Check sheet for the modelled part. Datum: model origin and axes. Units: mm. Face numbers are marked on the shaded views. A direction names the side the tool comes from. Give positions to 0.01 mm unless a question says otherwise; leave off trailing zeros. One line per item, written item: value. Start each with the question number.
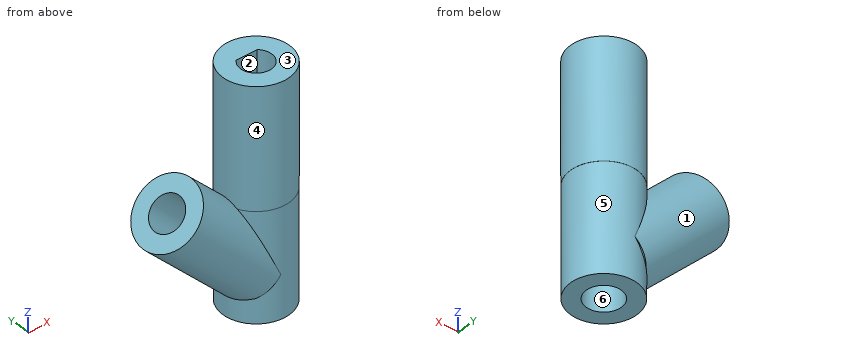
from build123d import *

# Parameters (mm, degrees)
SKETCH841_R     = 5.575015
PAD364_DEPTH    = 20
SKETCH842_R     = 5.560307
PAD365_DEPTH    = 18
SKETCH843_R     = 5.579276
PAD366_DEPTH    = 20
SKETCH844_R     = 2.85
POCKET224_DEPTH = 20
SKETCH845_R     = 2.95
POCKET225_DEPTH = 18.001


with BuildPart() as part:
    # Sketch841 → Pad364 (new body)
    with BuildSketch(Plane.XY):
        Circle(SKETCH841_R)
        with BuildLine():
            ThreePointArc((-1.794436, 1.881489), (0, -2.6), (1.794436, 1.881489))
            Line((-1.794436, 1.881489), (1.794436, 1.881489))
        make_face(mode=Mode.SUBTRACT)
    extrude(amount=PAD364_DEPTH)

    # Sketch842 → Pad365 (join)
    with BuildSketch(Plane.XY):
        Circle(SKETCH842_R)
    extrude(amount=-PAD365_DEPTH)

    # Sketch843 → Pad366 (join)
    with BuildSketch(Plane(origin=(-9, 0, 9), x_dir=(0.707107, 0, 0.707107), z_dir=(-0.707107, 0, 0.707107))):
        with Locations((-8.742249, 0)):
            Circle(SKETCH843_R)
    extrude(amount=-PAD366_DEPTH)

    # Sketch844 → Pocket224 (cut)
    with BuildSketch(Plane(origin=(-9, 0, 9), x_dir=(0.707107, 0, 0.707107), z_dir=(-0.707107, 0, 0.707107))):
        with Locations((-8.742247, 0)):
            Circle(SKETCH844_R)
    extrude(amount=-POCKET224_DEPTH, mode=Mode.SUBTRACT)

    # Sketch845 → Pocket225 (cut, through all)
    with BuildSketch(Plane.XY):
        Circle(SKETCH845_R)
    extrude(amount=-POCKET225_DEPTH, mode=Mode.SUBTRACT)


with BuildPart() as part_1:
    # Body064 placement: moved
    add(part.part.moved(Location((-52, -108, 0))))


solid = part_1.part
1) Cross-section at B-B (y = -108.5). State how many separate pieces and enclosed holes the cut face has, plus the area to 3 significant figures.
2) Gauge pin test, flat ends, axial feed: pin 1 (5.5 mm diameter, centred on x = -52, y = -108, fed in from -Z); pin 2 (1.5 mm diameter, centred on x = -60.5, z = -9, fed in from -Y); pin 3 (1 mm diameter, centred on x = -67, z = -1, fed in from -Y). Record the tip position at first contact, or that the pin passes through.
3) Draft check along Y on the marked faces 1, 2 and 3. Enter one of: released by +Y, released by -Y, zero draft, split by the parting line, or undercut.
4) Tool access check on the marked faces 4, 5 and 6. Record the directions out of +Z, -Z, +X, -X, +Y, -Y that give a thin tool (end or side, any length) a straight path to the whole face; none if there is none.
5) Material ranges on L1, parallel to Y at x = -52, z = -5; L2, parallel to X at y = -108, z = 9; L3, parallel to Y at x = -63.75, z = 2, recorded low to high. Write a range as from..to.
Data:
1. separate pieces: 3
1. enclosed holes: 0
1. area: 269 mm2
2. pin 1: stops at z = 0
2. pin 2: stops at y = -112.78
2. pin 3: stops at y = -113.18
3. face 1: split by the parting line
3. face 2: undercut
3. face 3: zero draft
4. face 4: +Z
4. face 5: none
4. face 6: -Z
5. L1: y = -113.56..-110.95, -105.05..-102.44
5. L2: x = -57.58..-54.6, -49.4..-46.42
5. L3: y = -113.26..-110.17, -105.83..-102.74
